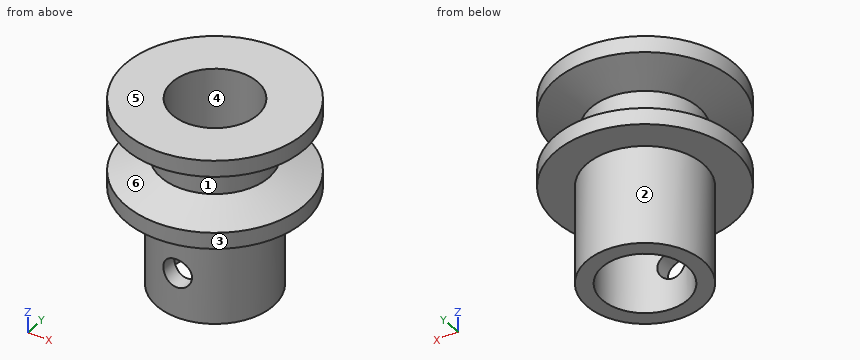
```python
from build123d import *

# Parameters (mm, degrees)
CROQUIS7_R            = 3.175
CORTAR_EXTRUIR2_DEPTH = 21


with BuildPart() as part:
    # Croquis2 → Revolución2 (revolve)
    with BuildSketch(Plane(origin=(0, 0, 0), x_dir=(1, 0, 0), z_dir=(0, 1, 0))):
        Polygon((20, 0), (20, 3.65), (12.0625, 6.825), (12.0625, 13.175), (20, 16.35), (20, 20), (13, 20), (13, 42), (9.525, 42), (9.525, 0), align=None)
    revolve(axis=Axis((0, 0, 0), (0, 0, -1)))

    # Croquis7 → Cortar-Extruir2 (cut, through all)
    with BuildSketch(Plane(origin=(0, 0, 0), x_dir=(1, 0, 0), z_dir=(0, 1, 0))):
        with Locations((0, 32)):
            Circle(CROQUIS7_R)
    extrude(amount=-CORTAR_EXTRUIR2_DEPTH, mode=Mode.SUBTRACT)


solid = part.part
```
Verification items for the finished model (mm, model axes). Face numbers are marked on the shaded views. A direction names the side the tool comes from. Coordinates: 2 decimals unless noted, no trailing zeros. Order: outer loops, then holes, each group sorted by start corner. A loop starts at its lowest first (then second) coordinate and runs counter-clockwise, first axis right, second up. Notation, with made-up numbers: (55, 79.25) -> (114, 79.25) arc R34 ccw to (114, 114.25) -> close; hole circle Ø3 at (38.25, -15.5). An arc over 180 degrees is marked (long way). Put each result on its own line as item: value. Start each with the question number.
1) Material ranges on L1, parallel to Z at x = 0, y = -10.3 (3 decimals); L2, parallel to Y at x = 0, z = -9 (1 decimal); L3, parallel to X at y = 5, z = -35, recorded low to high.
2) Go/stop test with flat-tipped pins: pin 1 (12 mm diameter, centred on x = -3.5, y = -5.5, fed in from +Z); pin 2 (8 mm diameter, centred on x = 4, z = -15.5, fed in from -Y); pin 3 (5 mm diameter, centred on x = -10.5, z = -16, fed in from +Y); pin 4 (6 mm diameter, centred on y = 8.5, z = -32.5, fed in from +X). Record where each tip stops, or that it passes through.
3) Cross-section at A-A (x = 0). State how many separate pieces and enclosed holes the cut face has, plus the area to 3 significant figures.
4) Cross-section at D-D (z = -24). Enter the section's corners in (x, y) (3 decimals).
5) Tool access check on the marked faces 1, 2 and 3. Record the directions out of +Z, -Z, +X, -X, +Y, -Y that give a thin tool (end or side, any length) a straight path to the whole face; none if there is none.
6) Release check for a two-part mould opening along X. For the marked faces 4, 5 and 6 record: pulls with the +X half, pulls with the -X half, needs draft (parallel to the pull), parting line crosses it, or undercut.
Geometry check:
1. L1: z = -42 to -35.175, -28.825 to 0
1. L2: y = -12.1 to -9.5, 9.5 to 12.1
1. L3: x = -12 to -8.11, 8.11 to 12
2. pin 1: stops at z = 0
2. pin 2: stops at y = -20
2. pin 3: stops at y = 18.32
2. pin 4: stops at x = 11.78
3. separate pieces: 3
3. enclosed holes: 0
3. area: 399 mm^2
4. outline: circle Ø26 at (0, 0); hole circle Ø19.05 at (0, 0)
5. face 1: none
5. face 2: -Z
5. face 3: +Z, -Z
6. face 4: undercut
6. face 5: needs draft
6. face 6: parting line crosses it
